The drawing under review shows one solid part. Ordinate dimensions are in mm from its lowest x, y, z. A direction names the side the tool comes from. Give positions to 0.01 mm unless a question says otherwise; leave off trailing zeros. Write each loop counter-clockwise with the first axis right and the second up, starting at its lowest first coordinate (ties: lowest second). Pieces come first, ordered by that corner, then holes. Notation, with made-up numbers: M 67,88.25 L 123,88.25 A27 cw 123,112.25 Z; hole C 16,-37.5 d6. An arc over 180 degrees is marked long. Write each question's results on one line, items separated by ' | '. Start each with the question number.
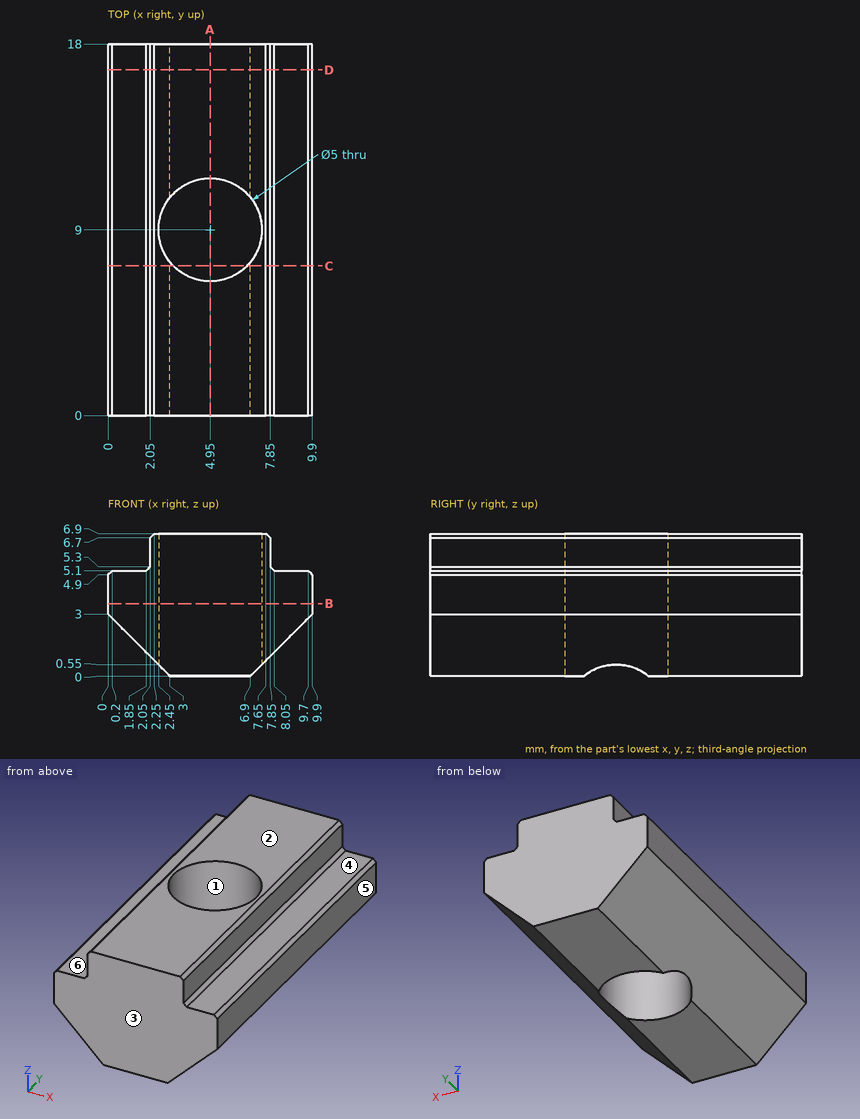
Q1. For the marked faces 4, 5 and 6, list the 3-axis set-ups (+Z, -Z, +X, -X, +Y, -Y) from which the entire face can be reached by the end or side of a thin tool; tool diameter is ignored.
Q2. Wall thickness on line 1 along Y through (x, z) = (4.95, 2.75); line 2 along X through (y, z) = (9, 4.25); line 3 along Y through (x, z) = (3.75, 4.75): over which ranges is each line inside the solid? List them lowest first. Write a range as from..to.
Q3. We need section D-D on y = 16.75. Write out the cut boundary in (x, z).
Q4. We need section C-C on y = 7.25. Write out the cut boundary in (x, z), and give its area (3 significant figures).
Q5. We need section A-A on x = 4.95. Write out the cut boundary in (y, z).
Q6. The part is to be moulded in two halves that separate along Y. For the marked faces 1, 2 and 3, say which applies: pulls with the +Y half, pulls with the -Y half, needs draft (parallel to the pull), parting line crosses it, or undercut.
Q7. We need section B-B on z = 3.5. Write out the cut boundary in (x, y), and give its area (3 significant figures).
Q8. For pin 1 Ø4 at (x, z) = (6, 5) entering from -Y; pin 2 Ø0.8 at (x, y) = (1, 11.5) entering from +Z; pin 3 Ø0.7 at (y, z) = (11, 6) entering from +X, all flat-tipped, find the tip position at first contact; note any pin that passes through.
Answer sheet:
1) face 4: +Z, +X, +Y, -Y | face 5: +Z, -Z, +X, +Y, -Y | face 6: +Z, -X, +Y, -Y
2) line 1: 0..6.5, 11.5..18 | line 2: 0..2.45, 7.45..9.9 | line 3: 0..6.81, 11.19..18
3) outline: M 0,3 L 3,0 L 6.9,0 L 9.9,3 L 9.9,4.9 L 9.7,5.1 L 8.05,5.1 L 7.85,5.3 L 7.85,6.7 L 7.65,6.9 L 2.25,6.9 L 2.05,6.7 L 2.05,5.3 L 1.85,5.1 L 0.2,5.1 L 0,4.9 Z
4) outline: M 0,3 L 3,0 L 3.16,0 L 3.16,6.9 L 2.25,6.9 L 2.05,6.7 L 2.05,5.3 L 1.85,5.1 L 0.2,5.1 L 0,4.9 Z; M 6.74,0 L 6.9,0 L 9.9,3 L 9.9,4.9 L 9.7,5.1 L 8.05,5.1 L 7.85,5.3 L 7.85,6.7 L 7.65,6.9 L 6.74,6.9 Z | area: 27.3 mm^2
5) outline: M 0,0 L 6.5,0 L 6.5,6.9 L 0,6.9 Z; M 11.5,0 L 18,0 L 18,6.9 L 11.5,6.9 Z
6) face 1: undercut | face 2: needs draft | face 3: pulls with the -Y half
7) outline: M 0,0 L 9.9,0 L 9.9,18 L 0,18 Z; hole C 4.95,9 d5 | area: 159 mm^2
8) pin 1: y = 0 | pin 2: z = 5.1 | pin 3: x = 7.85
